from build123d import *

# Parameters (mm, degrees)
F1_DEPTH    = 12
F2_W        = 6
F2_H        = 22.400515154
F4_DEPTH    = 1
F6_D        = 2.5
F6_DEPTH    = 9.5
F6_TIP      = 0.7510757738
F7_R        = 0.5
F8_T1_DEPTH = 4.7928932188
F8_T3_DEPTH = 6.7426406871
F9_R        = 0.5


# Not quite as in the source:
# - a fillet or chamfer that OpenCascade refuses, or shapes differently, is made with other operations: its cross-section is extruded or revolved along the edge and cut away or added


with BuildPart() as f1:
    # F0 (on Front) → F1 (new body)
    with BuildSketch(Plane.XZ):
        Polygon((0, 14.5), (0, 0), (10, 0), (10, 14.5), (6.5, 18), (3.5, 18), align=None)
    extrude(amount=F1_DEPTH)

    # F2 (on face) → F4 (cut)
    with BuildSketch(Plane.XZ.offset(12)):
        with Locations((5, 11.200257577)):
            Rectangle(F2_W, F2_H)
        Polygon((2, 16.5), (2, 0), (8, 0), (8, 16.5), (6.5, 18), (3.5, 18), align=None)
    extrude(amount=-F4_DEPTH, mode=Mode.SUBTRACT)

    # F6
    with Locations(Plane.XZ.offset(12)):
        with Locations((4.8096684931, 13.5), (5, 4.5)):
            Hole(F6_D / 2, depth=F6_DEPTH)
            with Locations((0, 0, -(F6_DEPTH + F6_TIP / 2))):  # 118° drill point
                Cone(0, F6_D / 2, F6_TIP, mode=Mode.SUBTRACT)

    # F7
    f7_edges = [f1.edges().sort_by_distance(p)[0] for p in [
        (10, 0, 7.25),
        (8.25, 0, 16.25),
        (0, 0, 7.25),
        (5, 0, 0),
    ]]
    fillet(f7_edges, radius=F7_R)

    # F8: fillet of radius 0.5 on 2 edges, made by hand

    # F8_s2 → F8_t1 (cut)
    with BuildSketch(Plane.YZ.offset(2.25)):
        with BuildLine():
            ThreePointArc((0, 17.5), (-0.1464466094, 17.8535533906), (-0.5, 18))
            Line((-0.5, 18), (0, 18))
            Line((0, 18), (0, 17.5))
        make_face()
    extrude(amount=F8_T1_DEPTH, mode=Mode.SUBTRACT)

    # F8_s4 → F8_t3 (cut)
    with BuildSketch(Plane(origin=(11.6338834765, 0, 11.6338834765), x_dir=(0, 1, 0), z_dir=(-0.7071067812, 0, -0.7071067812))):
        with BuildLine():
            ThreePointArc((-0.5, -10.2530483272), (-0.1464466094, -10.1066017178), (0, -9.7530483272))
            Line((0, -9.7530483272), (0, -10.2530483272))
            Line((0, -10.2530483272), (-0.5, -10.2530483272))
        make_face()
    extrude(amount=F8_T3_DEPTH, mode=Mode.SUBTRACT)

    # F9
    f9_edges = [f1.edges().sort_by_distance(p)[0] for p in [
        (3.5, -5.75, 18),
        (0, -6.25, 14.5),
        (6.5, -5.75, 18),
    ]]
    fillet(f9_edges, radius=F9_R)


solid = f1.part
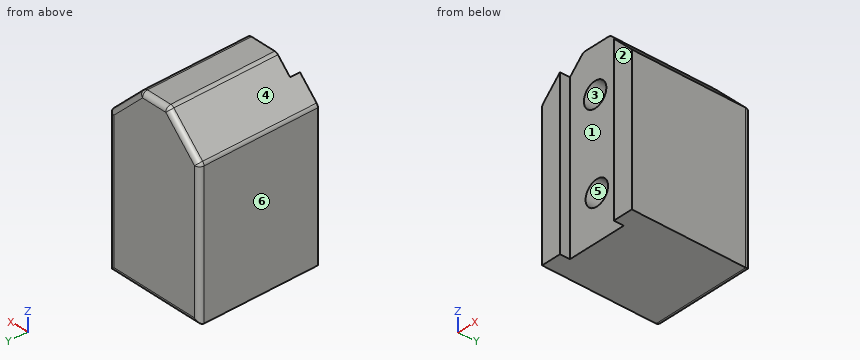
CAD build for the part. Positions are in the model's coordinates, mm. Face numbers are marked on the shaded views. A direction names the side the tool comes from. Coordinates: 2 decimals unless noted, no trailing zeros. Write each loop counter-clockwise with the first axis right and the second up, starting at its lowest first coordinate (ties: lowest second). Pieces come first, ordered by that corner, then holes. Notation, with made-up numbers: M -7,-2 L 39,-2 A34 ccw 39,28 Z; hole C -5,57.5 d3. An arc over 180 degrees is marked long. Answer as a JSON object with one key per item and string values. Group by question number.
1) Mould opens along Z. For the marked faces 4, 5 and 6 say: +Z half, -Z half, draft (parallel to the pull), parting line (faces both ways), or undercut.
2) Saw through at A-A (z = 11.75). Write the cut outline in (x, y).
3) Tool access for the marked faces 1, 2 and 3: list every direction of +Z, -Z, +X, -X, +Y, -Y with a clear straight run to the whole face (end or side of a thin tool).
4) Pin check, flat tip, straight feed: pin 1 Ø3 at (x, z) = (4, 7) entering from -Y. Stop position of the tip, or through.
5) Wall check: line 1 (Z direction, x = 5, y = -4.5); line 2 (X direction, y = -6.5, z = 4.5); line 3 (Y direction, x = 4, z = 7.25). Give the ranges that are in metal, low to high. Write a range as from..to.
6) Saw through at B-B (y = -9.25). Write the cut outline in (x, z).
Values follow:
{
 "1": {"face 4": "+Z half", "face 5": "undercut", "face 6": "draft"},
 "2": {"outline": "M 0,-12 L 2,-12 L 2,-11 L 8,-11 L 8,-12 L 10,-12 L 10,-0.5 A0.5 ccw 9.5,0 L 0.5,0 A0.5 ccw 0,-0.5 Z"},
 "3": {"face 1": "+Z, -Z, -Y", "face 2": "+Z, -Z, +X, -X, -Y", "face 3": "-Y"},
 "4": {"pin 1": "stops at y = -11"},
 "5": {"line 1": "z = 0..3.25, 5.75..12.26, 14.74..18", "line 2": "x = 0..3.75, 6.25..10", "line 3": "y = -11..0"},
 "6": {"outline": "M 0,0 L 10,0 L 10,14.5 L 6.65,17.85 A0.5 ccw 6.29,18 L 3.71,18 A0.5 ccw 3.35,17.85 L 0.15,14.65 A0.5 ccw 0,14.29 Z; hole C 4.81,13.5 d2.5; hole C 5,4.5 d2.5"}
}
